Autodesk Inventor part; units mm, degrees
ref_plane "YZ Plane" through (0, 0, 0) normal (1, 0, 0) x (0, 1, 0)
ref_plane "XZ Plane" through (0, 0, 0) normal (0, 1, 0) x (-1, 0, 0)
ref_plane "XY Plane" through (0, 0, 0) normal (0, 0, 1) x (1, 0, 0)
sketch "Sketch1" plane through (0, 0, 0) normal (0, 0, 1) x (1, 0, 0)
  circle A0 centre (0, 0) radius 14
  line L0 (-26, -20) -> (26, -20)
  line L1 (26, -20) -> (26, 8)
  line L2 (26, 8) -> (14, 20)
  line L3 (14, 20) -> (-14, 20)
  line L4 (-14, 20) -> (-26, 8)
  line L5 (-26, 8) -> (-26, -20)
  circle A1 centre (0, 0) radius 19 construction
  circle A2 centre (13.435, 13.435) radius 2.5
  circle A3 centre (-13.435, -13.435) radius 2.5
  circle A4 centre (13.435, -13.435) radius 2.5
  circle A5 centre (-13.435, 13.435) radius 2.5
  circle A6 centre (-19, 0) radius 2.5
  circle A7 centre (19, 0) radius 2.5
  line L6 (-13.435, 13.435) -> (0, 0) construction
  line L7 (0, 0) -> (-19, 0) construction
  point P0 (0, 20)
  point P1 (0, -20)
  dimension "d0" = 28
  dimension "d1" = 40
  dimension "d2" = 52
  dimension "d3" = 38
  dimension "d4" = 5
  dimension "d5" = 45
  dimension "d6" = 20
  dimension "d7" = 135
  dimension "d8" = 12
extrude "Extrusion1" add sketch "Sketch1" along normal blind 40
sketch "Sketch2" plane through (-26, -20, 0) normal (0, -1, 0) x (1, 0, 0)
  circle A0 centre (6, 32) radius 2.5
  circle A1 centre (46, 32) radius 2.5
  circle A2 centre (6, 8) radius 2.5
  circle A3 centre (46, 8) radius 2.5
  line L0 (6, 32) -> (46, 32) construction
  line L1 (46, 32) -> (46, 8) construction
  line L2 (46, 8) -> (6, 8) construction
  line L3 (6, 8) -> (6, 32) construction
  line L4 (0, 40) -> (52, 40) construction
  line L5 (52, 0) -> (52, 40) construction
  point P0 (26, 0)
  point P1 (26, 32)
  point P2 (26, 40)
  point P3 (46, 20)
  point P4 (52, 20)
  dimension "d11" = 5
  dimension "d12" = 40
  dimension "d13" = 24
extrude "Extrusion2" cut sketch "Sketch2" against normal blind 10
properties part number "DSG16H"
Build history of the part. All positions in model axes, mm. A direction names the side the tool comes from. Coordinates: 2 decimals unless noted, no trailing zeros. Order: outer loops, then holes, each group sorted by start corner. A loop starts at its lowest first (then second) coordinate and runs counter-clockwise, first axis right, second up. Notation, with made-up numbers: (15.5, -17) -> (54.5, -17) arc R28 ccw to (54.5, 19) -> close; hole circle Ø6 at (0, 80.25). An arc over 180 degrees is marked (long way). Answer in a Markdown table with one row per item. Add a question column.
Q1. Band-saw the part on D-D, the plane z = 3. List the corners of the cut face in (x, y) (3 decimals), then the cut area to 3 significant figures.
Q2. Wall check: line 1 along Z through (x, y) = (-20, -12); line 2 along X through (y, z) = (13, 7); line 3 along X through (y, z) = (-15.5, 2). Give the ranges that are in metal, low to high. Write a range as [from, to].
Q3. Band-saw the part on B-B, the plane x = 18.5. List the corners of the cut face in (y, z), then the cut area to 3 significant figures.
Q4. Band-saw the part on A-A, the plane y = 0. List the corners of the cut face in (x, z).
Q5. Drop flat-ended pins along their axis: pin 1 (2.5 mm diameter, centred on x = -21, z = 32.5, fed in from -Y); pin 2 (3 mm diameter, centred on x = -20, z = 8, fed in from +Y); pin 3 (3 mm diameter, centred on x = 13.435, y = -13.435, fed in from +Z). Give the stop position or say it passes through.
Q6. Band-saw the part on C-C, the plane y = -15. List the corners of the cut face in (x, z).
Q7. Mould opens along X. For faces 1 (the face through (18.16, -15.07, 33.69)), 2 (the face through (0, -20, 20)), 3 (the face through (-26, -6, 20)) say: +X half, -X half, draft (parallel to the pull), parting line (faces both ways), or undercut.
Q8. Which spindle directions (+Z, -Z, +X, -X, +Y, -Y) get a long thin tool onto all of the face, cutting with end or side? Do faces 4 (the face through (12.932, 5.362, 19.72)), 5 (the face through (20, -10, 32)). Say none if no direction does.
Answers follow:
| question | item | result |
|---|---|---|
| 1 | outline | (-26, -20) -> (26, -20) -> (26, 8) -> (14, 20) -> (-14, 20) -> (-26, 8) -> close; hole circle Ø5 at (-19, 0); hole circle Ø5 at (-13.435, -13.435); hole circle Ø5 at (-13.435, 13.435); hole circle Ø28 at (0, 0); hole circle Ø5 at (13.435, -13.435); hole circle Ø5 at (13.435, 13.435); hole circle Ø5 at (19, 0) |
| 1 | area | 1,200 mm^2 |
| 2 | line 1 | [0, 5.5], [10.5, 29.5], [34.5, 40] |
| 2 | line 2 | [-21, -15.9], [-10.97, -5.2], [5.2, 10.97], [15.9, 21] |
| 2 | line 3 | [-26, -14.84], [-12.03, 12.03], [14.84, 26] |
| 3 | outline | (-20, 0) -> (-2.45, 0) -> (-2.45, 40) -> (-20, 40) -> (-20, 34) -> (-10, 34) -> (-10, 30) -> (-20, 30) -> (-20, 10) -> (-10, 10) -> (-10, 6) -> (-20, 6) -> close; (2.45, 0) -> (15.5, 0) -> (15.5, 40) -> (2.45, 40) -> close |
| 3 | area | 1,140 mm^2 |
| 4 | outline | (-26, 0) -> (-21.5, 0) -> (-21.5, 40) -> (-26, 40) -> close; (-16.5, 0) -> (-14, 0) -> (-14, 40) -> (-16.5, 40) -> close; (14, 0) -> (16.5, 0) -> (16.5, 40) -> (14, 40) -> close; (21.5, 0) -> (26, 0) -> (26, 40) -> (21.5, 40) -> close |
| 5 | pin 1 | y = -10 |
| 5 | pin 2 | y = 15.5 |
| 5 | pin 3 | through |
| 6 | outline | (-26, 0) -> (-15.38, 0) -> (-15.38, 40) -> (-26, 40) -> close; (-11.49, 0) -> (11.49, 0) -> (11.49, 40) -> (-11.49, 40) -> close; (15.38, 0) -> (26, 0) -> (26, 40) -> (15.38, 40) -> close; hole circle Ø5 at (-20, 8); hole circle Ø5 at (-20, 32); hole circle Ø5 at (20, 8); hole circle Ø5 at (20, 32) |
| 7 | face 1 | undercut |
| 7 | face 2 | draft |
| 7 | face 3 | -X half |
| 8 | face 4 | +Z, -Z |
| 8 | face 5 | -Y |
